from build123d import *

# Parameters (mm, degrees)
SKETCH_1_W          = 45.7
SKETCH_1_H          = 24
EXTRUDE_1_DEPTH     = 9.4
SKETCH_2_R          = 1.75
CUT_EXTRUDE_1_DEPTH = 6
SKETCH_3_R          = 4
EXTRUDE_2_DEPTH     = 7.6
EXTRUDE_3_DEPTH     = 8
FILLET_1_R          = 10
CHAMFER_1_SIZE      = 1.5
SKETCH_5_R          = 3.5
EXTRUDE_4_DEPTH     = 8
EXTRUDE_4_TAPER     = 5
FILLET_2_R          = 1


with BuildPart() as part:
    # 草图1 → 凸台-拉伸1 (new body)
    with BuildSketch(Plane(origin=(0, 0, 0), x_dir=(1, 0, 0), z_dir=(0, 1, 0))):
        Rectangle(SKETCH_1_W, SKETCH_1_H)
    extrude(amount=EXTRUDE_1_DEPTH)

    # 草图2 → 切除-拉伸1 (cut)
    with BuildSketch(Plane(origin=(22.85, 0, 0), x_dir=(0, 0, -1), z_dir=(1, 0, 0))):
        with Locations((-7.5, 5)):
            Circle(SKETCH_2_R)
        with Locations((0, 5)):
            Circle(SKETCH_2_R)
        with Locations((7.5, 5)):
            Circle(SKETCH_2_R)
    extrude(amount=-CUT_EXTRUDE_1_DEPTH, mode=Mode.SUBTRACT)

    # 草图3 → 凸台-拉伸2 (add)
    with BuildSketch(Plane.ZY.offset(22.85)):
        with Locations(Location((7, 5, 0), (0, 0, 180))):
            Circle(SKETCH_3_R)
    extrude(amount=EXTRUDE_2_DEPTH)

    # 草图4 → 凸台-拉伸3 (add)
    with BuildSketch(Plane.ZY.offset(22.85)):
        Polygon((4.3, 11.5), (9.7, 11.5), (12, 9.4), (2, 9.4), align=None)
    extrude(amount=-EXTRUDE_3_DEPTH)

    # 圆角1
    # the kernel refuses this fillet: 10 mm, written as the material it takes off along each edge
    with BuildSketch(Plane(origin=(-14.85, 11.5, -11.027671056), x_dir=(-1, 0, 0), z_dir=(0, 0, 1))) as fillet_1_piece_1:
        with BuildLine():
            CenterArc((6.131068422, 10), FILLET_1_R, 232.185511494, 37.814488506)
            Line((0, 2.1), (0, 0))
            Line((0, 0), (6.131068422, 0))
        make_face()
    extrude(amount=36.055342112, mode=Mode.SUBTRACT)

    # 倒角1
    # the kernel refuses this chamfer: 1.5 mm, written as the material it takes off along each edge
    with BuildSketch(Plane(origin=(-18.707524482, 9.4, 12), x_dir=(0, -1, 0), z_dir=(1, 0, 0))) as chamfer_1_piece_1_section:
        Polygon((CHAMFER_1_SIZE, 0), (0, CHAMFER_1_SIZE), (0, 0), align=None)
    chamfer_1_piece_1 = extrude(amount=45.415048964, mode=Mode.PRIVATE)
    chamfer_1_piece_1 = chamfer_1_piece_1 - Plane(origin=(-20.981068422, 1.5, 12), x_dir=(-1, 0, 0), z_dir=(0, 0, -1)) * Cylinder(10, 97, mode=Mode.PRIVATE)
    add(chamfer_1_piece_1, mode=Mode.SUBTRACT)
    with BuildSketch(Plane(origin=(-26.707524482, 0, 12), x_dir=(0, 1, 0), z_dir=(1, 0, 0)), Plane(origin=(26.707524482, 9.4, -12), x_dir=(0, 0, 1), z_dir=(-1, 0, 0))) as chamfer_1_piece_2:
        Polygon((CHAMFER_1_SIZE, 0), (0, -CHAMFER_1_SIZE), (0, 0), align=None)
    extrude(amount=53.415048964, mode=Mode.SUBTRACT)
    with BuildSketch(Plane(origin=(26.707524482, 0, -12), x_dir=(0, 0, 1), z_dir=(-1, 0, 0))) as chamfer_1_piece_3:
        Polygon((CHAMFER_1_SIZE, 0), (0, CHAMFER_1_SIZE), (0, 0), align=None)
    extrude(amount=53.415048964, mode=Mode.SUBTRACT)

    # 草图5 → 凸台-拉伸4 (add)
    with BuildSketch(Plane.ZY.offset(22.85)):
        with Locations((-7, 5)):
            Circle(SKETCH_5_R)
    extrude(amount=EXTRUDE_4_DEPTH, taper=EXTRUDE_4_TAPER)

    # 圆角2
    fillet_2_edges = [part.edges().sort_by_distance(p)[0] for p in [
        (-30.45, 5, 11),
    ]]
    fillet(fillet_2_edges, radius=FILLET_2_R)


solid = part.part
Could you check a few things on this model? Use its own coordinates, in mm. A direction names the side the tool comes from. Give positions to 0.01 mm unless a question says otherwise; leave off trailing zeros. Write each loop counter-clockwise with the first axis right and the second up, starting at its lowest first coordinate (ties: lowest second). Pieces come first, ordered by that corner, then holes. Notation, with made-up numbers: (-29, 34.5) -> (28, 34.5) arc R13 ccw to (28, 39.5) -> close; hole circle Ø6 at (63, 20). An arc over 180 degrees is marked (long way). Write each question's results on one line, items separated by ' | '. Start each with the question number.
Q1. Suppose I cut it at B-B, the plane z = 0. List the corners of the cut face in (x, y) for me, and give its area (3 significant figures).
Q2. Suppose I cut it at C-C, the plane x = -26. List the corners of the cut face in (y, z) for me, and give its area (3 significant figures).
Q3. I'm going to push flat-ended pins straight in: pin 1 Ø5 at (y, z) = (4.5, 7.5) entering from -X; pin 2 Ø3 at (y, z) = (5, 0) entering from -X; pin 3 Ø1 at (x, z) = (-20.5, -7.5) entering from +Y. Where does each tip first touch, or does it pass through?
Q4. I need wall thicknesses on probe 1 along Y at (x, z) = (20.85, 0); probe 2 along X at (y, z) = (3.5, -6.75); probe 3 along Y at (x, z) = (-14, -6.5). Which ranges of each line are inside material? Lowest first, please.
Q5. Suppose I cut it at A-A, the plane x = -3.5. List the corners of the cut face in (y, z) for me, and give its area (3 significant figures).
Q6. We'd pull the mould along Z, two halves only. Please class faces 1 (the face through (-19.79, 10.23, 11.09)), 2 (the face through (0, 0, 0)), 3 (the face through (-22.85, 5, 0)): +Z half, -Z half, draft (parallel to the pull), parting line (faces both ways), or undercut.
Q7. Suppose I cut it at D-D, the plane y = 10. List the corners of the cut face in (x, z) for me, and give its area (3 significant figures).
Q8. Which directions (+Z, -Z, +X, -X, +Y, -Y) give clear straight access to the entire face, cutting with the end or side of a thin tool? Please do faces 4 (the face through (0, 9.4, 0)), 5 (the face through (-0.3, 0.8, 11.3)), 6 (the face through (-26.1, 7.4, 10.2)), 7 (the face through (-22, 11.5, 7)), 8 (the face through (16.85, 5, -7)).
Outcome:
1) outline: (-22.85, 0) -> (22.85, 0) -> (22.85, 3.25) -> (16.85, 3.25) -> (16.85, 6.75) -> (22.85, 6.75) -> (22.85, 9.4) -> (-22.85, 9.4) -> close | area: 409 mm2
2) outline: circle Ø8 at (5, 7); circle Ø6.45 at (5, -7) | area: 82.9 mm2
3) pin 1: x = -30.45 | pin 2: x = -22.85 | pin 3: y = 9.4
4) probe 1: 0 to 3.25, 6.75 to 9.4 | probe 2: -30.85 to 16.85 | probe 3: 0 to 9.4
5) outline: (0, -10.5) -> (1.5, -12) -> (7.9, -12) -> (9.4, -10.5) -> (9.4, 10.5) -> (7.9, 12) -> (1.5, 12) -> (0, 10.5) -> close | area: 221 mm2
6) face 1: +Z half | face 2: draft | face 3: undercut
7) outline: (-22.85, 2.66) -> (-15.71, 2.66) -> (-15.71, 11.34) -> (-22.85, 11.34) -> close | area: 62.0 mm2
8) face 4: -Z, +X, +Y | face 5: +Z, +X, -X, -Y | face 6: -X | face 7: +Z, -Z, +X, -X, +Y | face 8: +X
